Model file for the job. Use its own axes, mm. Face numbers are marked on the shaded views. Coordinates: 2 decimals unless noted, no trailing zeros. Write each loop counter-clockwise with the first axis right and the second up, starting at its lowest first coordinate (ties: lowest second). Pieces come first, ordered by that corner, then holes. Notation, with made-up numbers: M -29,45 L 13,45 A21 ccw 13,49 Z; hole C -17.5,30.5 d5. An arc over 180 degrees is marked long. One line per question, with ' | ' between items. Start each with the question number.
(1) Wall check: probe 1 along Y at (x, z) = (0, 5.75); probe 2 along Y at (x, z) = (78, 5.25); probe 3 along X at (y, z) = (1.5, 2.75). Give the ranges that are in metal, low to high.
(2) Flat gauge pins, fed straight in: pin 1 Ø3 at (y, z) = (9, 3.5) entering from -X; pin 2 Ø2 at (x, z) = (-1, 3.5) entering from +Y; pin 3 Ø2 at (x, z) = (77, 6) entering from -Y. Where does each tip first touch, or does it go through?
(3) Two-plate mould, pull along Y, no slides. Class the marked faces 1 and 2: +Y half, -Y half, draft (parallel to the pull), parting line (faces both ways), or undercut.
(4) Cut at C-C (y = 0). Write the cut outline in (x, z), plus the area to 3 significant figures.
(5) Cut at B-B (z = 2). Write the cut outline in (x, y).
(6) Cut at A-A (x = 0). Write the cut outline in (y, z).
from build123d import *

# Parameters (mm, degrees)
SKETCH_R        = 70
SKETCH_R_2      = 2.5
PAD_DEPTH       = 10
CHAMFER_SIZE    = 1
CHAMFER001_SIZE = 0.5


with BuildPart() as part:
    # Sketch → Pad (new body)
    with BuildSketch(Plane.XY):
        with BuildLine():
            ThreePointArc((73.830888, 5), (-74, 0), (73.830888, -5))
            Line((78, -5), (73.830888, -5))
            ThreePointArc((78, -5), (83, 0), (78, 5))
            Line((73.830888, 5), (78, 5))
        make_face()
        Circle(SKETCH_R, mode=Mode.SUBTRACT)
        with Locations((78, 0)):
            Circle(SKETCH_R_2, mode=Mode.SUBTRACT)
    extrude(amount=PAD_DEPTH)

    # Chamfer
    chamfer_edges = [part.edges().sort_by_distance(p)[0] for p in [
        (-70, 0, 10),
    ]]
    chamfer(chamfer_edges, length=CHAMFER_SIZE)

    # Chamfer001
    chamfer001_edges = [part.edges().sort_by_distance(p)[0] for p in [
        (75.5, 0, 10),
    ]]
    chamfer(chamfer001_edges, length=CHAMFER001_SIZE)


solid = part.part
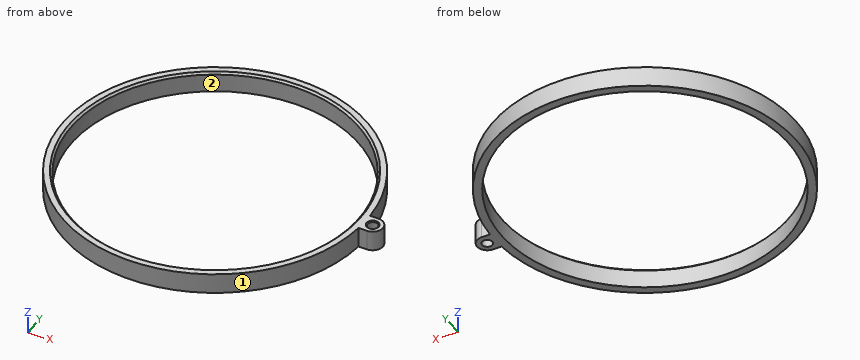
Filled in:
1) probe 1: -74 to -70, 70 to 74 | probe 2: -5 to -2.5, 2.5 to 5 | probe 3: -73.98 to -69.98, 69.98 to 76, 80 to 82.77
2) pin 1: x = -73.62 | pin 2: y = 74 | pin 3: y = -5
3) face 1: parting line | face 2: undercut
4) outline: M -74,0 L -70,0 L -70,9 L -71,10 L -74,10 Z; M 70,0 L 75.5,0 L 75.5,9.5 L 75,10 L 71,10 L 70,9 Z; M 80.5,0 L 83,0 L 83,10 L 81,10 L 80.5,9.5 Z | area: 119 mm²
5) outline: M 73.83,-5 L 78,-5 A5 ccw 78,5 L 73.83,5 A74 ccw long Z; hole C 0,0 d140; hole C 78,0 d5
6) outline: M -74,0 L -70,0 L -70,9 L -71,10 L -74,10 Z; M 70,0 L 74,0 L 74,10 L 71,10 L 70,9 Z
